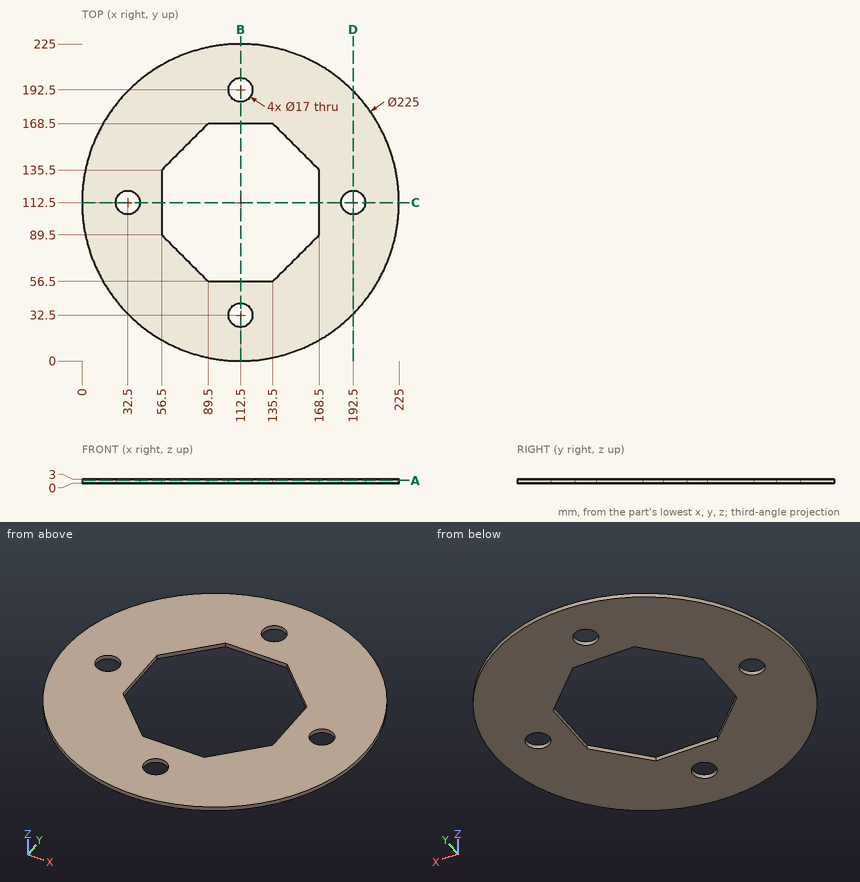
Verification items for this drawing (mm, ordinates from the low corner). Coordinates: 2 decimals unless noted, no trailing zeros. Loops run counter-clockwise (first coordinate to the right, second up) from the corner with the lowest first, then second, coordinate; pieces in that order, holes last. Notation, with made-up numbers: (74.5, -27) - (92.5, -27) arc R21 ccw to (92.5, -21) - close; hole circle Ø8 at (-28, 38.5). An arc over 180 degrees is marked (long way). One line per item, written item: value. Start each with the question number.
(1) Depth check by flat-ended pin: P1, Ø1.5, axis at x = 122.5, z = 1.5, coming from the -Y side; P2, Ø0.9, axis at y = 111.5, z = 1.5, coming from the +X side; P3, Ø1, axis at x = 162, z = 1, coming from the +Y side; P4, Ø2, axis at x = 164, y = 50, coming from the -Z side. Enter the tip coordinate at first touch or a pass-through.
(2) Cross-section at B-B on x = 112.5. Enter the section's corners in (y, z).
(3) Material ranges on line 1 (Y direction, x = 112.5, z = 1.5); line 2 (X direction, y = 185.5, z = 1.55); line 3 (X direction, y = 136.5, z = 0.65), recorded low to high. Write a range as [from, to].
(4) Cross-section at D-D on x = 192.5. Enter the section's corners in (y, z).
(5) Cross-section at A-A on z = 2.1. Enter the section's corners in (x, y).
Results below:
1. P1: stops at y = 0.38
1. P2: stops at x = 225
1. P3: stops at y = 213.77
1. P4: stops at z = 0
2. outline: (0, 0) - (24, 0) - (24, 3) - (0, 3) - close; (41, 0) - (56.5, 0) - (56.5, 3) - (41, 3) - close; (168.5, 0) - (184, 0) - (184, 3) - (168.5, 3) - close; (201, 0) - (225, 0) - (225, 3) - (201, 3) - close
3. line 1: y = [0, 24], [41, 56.5], [168.5, 184], [201, 225]
3. line 2: x = [26.9, 107.68], [117.32, 198.1]
3. line 3: x = [2.59, 57.5], [167.5, 222.41]
4. outline: (33.4, 0) - (104, 0) - (104, 3) - (33.4, 3) - close; (121, 0) - (191.6, 0) - (191.6, 3) - (121, 3) - close
5. outline: circle Ø225 at (112.5, 112.5); hole circle Ø17 at (32.5, 112.5); hole (56.5, 89.5) - (89.5, 56.5) - (135.5, 56.5) - (168.5, 89.5) - (168.5, 135.5) - (135.5, 168.5) - (89.5, 168.5) - (56.5, 135.5) - close; hole circle Ø17 at (112.5, 32.5); hole circle Ø17 at (112.5, 192.5); hole circle Ø17 at (192.5, 112.5)
